Read the model definition and answer for the solid it produces. Units are mm, in the model's axes. Face numbers are marked on the shaded views. Coordinates: 2 decimals unless noted, no trailing zeros. Loops run counter-clockwise (first coordinate to the right, second up) from the corner with the lowest first, then second, coordinate; pieces in that order, holes last. Notation, with made-up numbers: M 27.25,-19.5 L 46.25,-19.5 A7 ccw 46.25,-13.5 Z; hole C 14,-26 d10. An arc over 180 degrees is marked long. One line per item, written item: value. Start each with the question number.
1. The part is cut by section C-C (z = -8). Write down the section's boundary in (x, y) (1 decimal).
2. Determine the mould class of the marked faces 1, 2 and 3 for opening direction Y: +Y half, -Y half, draft (parallel to the pull), parting line (faces both ways), or undercut.
3. The part is cut by section A-A (y = 0). Write down the section's boundary in (x, z), then the cut area to 3 significant figures.
4. Consider probe 1 along Y at (x, z) = (0, -8.75); probe 2 along X at (y, z) = (-3.5, -9.75); probe 3 along Y at (x, z) = (-1, -8.5). Determine where each line is inside the solid, lowest interval first.
5. The part is cut by section D-D (z = 1.5). Write down the section's boundary in (x, y).
6. Flat-ended cylindrical pins translate along their axes: pin 1 (2 mm diameter, centred on y = -1, z = -6.5, fed in from +X); pin 2 (5 mm diameter, centred on x = 1.5, y = 1, fed in from -Z); pin 3 (2 mm diameter, centred on x = 3.5, y = 0, fed in from +Z); pin 4 (5 mm diameter, centred on y = -4.5, z = -1.5, fed in from +X). Find the tip coordinate at first contact, or state that the pin passes through.
Autodesk Inventor part; units mm, degrees
ref_plane "YZ Plane" through (0, 0, 0) normal (1, 0, 0) x (0, 1, 0)
ref_plane "XZ Plane" through (0, 0, 0) normal (0, 1, 0) x (-1, 0, 0)
ref_plane "XY Plane" through (0, 0, 0) normal (0, 0, 1) x (1, 0, 0)
sketch "RingSketch" plane through (0, 0, 0) normal (0, 0, 1) x (1, 0, 0)
  circle A0 centre (0, 0) radius 7
  dimension "RingDia" = 14
extrude "Ring" add sketch "RingSketch" against normal blind 1
sketch "ShankSketch" plane through (0, 0, -1) normal (0, 0, -1) x (-1, 0, 0)
  circle A0 centre (0, 0) radius 7
  dimension "ShankDia" = 14
extrude "Shank" add sketch "ShankSketch" along normal blind 10.536
sketch "ConeSketch" plane through (0, 0, 0) normal (1, 0, 0) x (0, 1, 0)
  line L0 (0, 0) -> (7, 0)
  line L1 (7, 0) -> (5, 3.4641)
  line L2 (5, 3.4641) -> (0, 3.4641)
  line L3 (0, 3.4641) -> (0, 0)
  line L4 (-7, 0) -> (7, 0)
  dimension "ConeAngle" = 60
  dimension "ConeBase" = 7
  dimension "ConeTipDia" = 5
revolve "Cone" add sketch "ConeSketch" angle 360 about axis through (0, 0, 3.4641) along (0, 0, -1)
sketch "SocketSketch" plane through (0, 0, 0) normal (0, 1, 0) x (-1, 0, 0)
  arc A0 (0, 0.4641) -> (0, 10.4641) centre (0, 5.4641) ccw
  line L0 (0, 10.4641) -> (0, 0.4641)
  line L1 (-5, 3.4641) -> (5, 3.4641)
  line L2 (5, 3.4641) -> (7, 0)
  point P0 (0, 0)
  dimension "RecessDia" = 10
  dimension "BallOffset" = 2
revolve "Socket" cut sketch "SocketSketch" angle 360 about axis through (0, 0, 10.4641) along (0, 0, -1)
sketch "MagnetHoleSketch" plane through (0, 0, -11.536) normal (0, 0, -1) x (-1, 0, 0)
  circle A0 centre (0, 0) radius 4.7625
  dimension "MagnetHoleDia" = 9.525
extrude "MagnetHole" cut sketch "MagnetHoleSketch" against normal blind 11.5001
sketch "PartLength" plane through (0, 0, 0) normal (0, 1, 0) x (-1, 0, 0)
  line L0 (-5, 3.4641) -> (5, 3.4641)
  line L1 (-7, -11.536) -> (7, -11.536)
  point P0 (0, 0)
  dimension "PartLen" = 15.0001
chamfer "Chamfer1" distance 1 angle 45 1 edges at (7, 0, -11.536)
equation "\"ShankDia\" = RingDia"
equation "\"ConeBase\" = 0.5 * RingDia"
equation "\"ConeTipDia\" = 0.5 * BallDia"
equation "\"RecessDia\" = BallDia"
properties part number "Rod End 9.5mm"
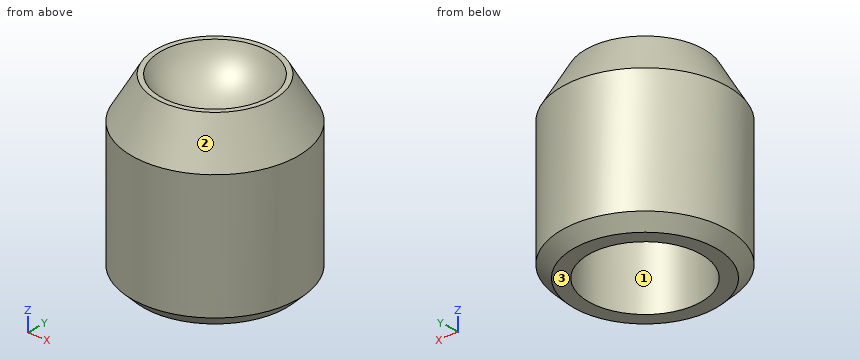
Answer block:
1. outline: C 0,0 d14; hole C 0,0 d9.5
2. face 1: undercut
2. face 2: parting line
2. face 3: draft
3. outline: M -7,-10.54 L -6,-11.54 L -4.76,-11.54 L -4.76,-0.04 L 4.76,-0.04 L 4.76,-11.54 L 6,-11.54 L 7,-10.54 L 7,0 L 5,3.46 L 4.58,3.46 A5 cw -4.58,3.46 L -5,3.46 L -7,0 Z
3. area: 72.7 mm2
4. probe 1: y = -7 to -4.76, 4.76 to 7
4. probe 2: x = -6.06 to -3.23, 3.23 to 6.06
4. probe 3: y = -6.93 to -4.66, 4.66 to 6.93
5. outline: C 0,0 d12.27; hole C 0,0 d6.09
6. pin 1: stops at x = 7
6. pin 2: stops at z = -0.04
6. pin 3: stops at z = 3.28
6. pin 4: stops at x = 6.71
